from build123d import *
from build123d.topology import SkipClean

# Parameters (mm, degrees)
SKETCH1_R           = 12.7
BOSS_EXTRUDE1_DEPTH = 5.08
BOSS_EXTRUDE2_START = 5.08
BOSS_EXTRUDE2_DEPTH = 5.08
BOSS_EXTRUDE3_DEPTH = 5.08


with BuildPart() as part:
    # Sketch1 → Boss-Extrude1 (new body)
    with BuildSketch(Plane.XY):
        Circle(SKETCH1_R)
    extrude(amount=BOSS_EXTRUDE1_DEPTH)

    # Sketch2 → Boss-Extrude2 (add)
    with SkipClean():  # the faces are left unmerged after this step: merging them gives an invalid solid
        with BuildSketch(Plane(origin=(0, 0, 0), x_dir=(-1, 0, 0), z_dir=(0, 0, -1)).offset(BOSS_EXTRUDE2_START)):
            with BuildLine():
                Line((12.296722124, 3.175), (-12.296722124, 3.175))
                ThreePointArc((-12.296722124, 3.175), (-12.7, 0), (-12.296722124, -3.175))
                Line((-12.296722124, -3.175), (12.296722124, -3.175))
                ThreePointArc((12.296722124, -3.175), (12.7, 0), (12.296722124, 3.175))
            make_face()
        extrude(amount=-BOSS_EXTRUDE2_DEPTH)

    # Sketch4 → Boss-Extrude3 (add)
    with SkipClean():  # the faces are left unmerged after this step: merging them gives an invalid solid
        with BuildSketch(Plane.XY.offset(5.08)):
            with BuildLine():
                Line((-3.175, -12.296722124), (-3.175, 12.296722124))
                ThreePointArc((-3.175, 12.296722124), (0, 12.7), (3.175, 12.296722124))
                Line((3.175, 12.296722124), (3.175, -12.296722124))
                ThreePointArc((3.175, -12.296722124), (0, -12.7), (-3.175, -12.296722124))
            make_face()
        extrude(amount=BOSS_EXTRUDE3_DEPTH)


solid = part.part
Verification items for the finished model (mm, model axes). A direction names the side the tool comes from. Round coordinates to 2 decimals unless told otherwise and drop trailing zeros. Order: outer loops, then holes, each group sorted by start corner. A loop starts at its lowest first (then second) coordinate and runs counter-clockwise, first axis right, second up.
1. Access from +Z, -Z, +X, -X, +Y, -Y to the whole of each face (thin tool, end or side, straight path). Record for faces 1 (the flat face through (0, -7, 0)), 2 (the flat face through (-7, 0, 5.08)), 3 (the flat face through (3.175, 0, 8)), 4 (the flat face through (0, 3.175, -3)).
Final values:
face 1: -Z, +X, -X, -Y
face 2: +Z, -X, +Y, -Y
face 3: +Z, +X, +Y, -Y
face 4: -Z, +X, -X, +Y
2. Go/stop test with flat-tipped pins: P1, Ø5.5, axis at y = -0.5, z = 7.5, coming from the -X side; P2, Ø1, axis at y = 9.5, z = 7, coming from the -X side (3 decimals); P3, Ø5, axis at y = 4.5, z = -2.5, coming from the -X side; P4, Ø1.5, axis at y = -3, z = 6.5, coming from the +X side (3 decimals). Record where each tip stops, or that it passes through.
Final values:
P1: stops at x = -12.7
P2: stops at x = -3.175
P3: stops at x = -12.54
P4: stops at x = 3.175
3. Section check A-A on x = 0. Record the cut outline in (y, z) (3 decimals), then the cut area to 3 significant figures.
Final values:
outline: (-12.7, 0) - (-3.175, 0) - (-3.175, -5.08) - (3.175, -5.08) - (3.175, 0) - (12.7, 0) - (12.7, 10.16) - (-12.7, 10.16) - close
area: 290 mm2
4. Section check B-B on y = 0. Record the cut outline in (x, z) (3 decimals), then the cut area to 3 significant figures.
Final values:
outline: (-12.7, -5.08) - (12.7, -5.08) - (12.7, 5.08) - (3.175, 5.08) - (3.175, 10.16) - (-3.175, 10.16) - (-3.175, 5.08) - (-12.7, 5.08) - close
area: 290 mm2
5. Thickness scan on L1, parallel to Z at x = -9, y = 3.5; L2, parallel to X at y = -3, z = 6.25 (3 decimals); L3, parallel to Z at x = 7.25, y = -3. Record the ranges inside material, lowest first.
Final values:
L1: z = 0 to 5.08
L2: x = -3.175 to 3.175
L3: z = -5.08 to 5.08
6. Section check C-C on z = 6.5. Record the cut outline in (x, y) (3 decimals), then the cut area to 3 significant figures.
Final values:
outline: (-3.175, -12.297) arc R12.7 ccw to (3.175, -12.297) - (3.175, 12.297) arc R12.7 ccw to (-3.175, 12.297) - close
area: 160 mm2
7. Section check D-D on z = 3.25. Record the cut outline in (x, y).
Final values:
outline: circle Ø25.4 at (0, 0)
